Can you work these out from the drawing? Everything is in mm from the part's minimum corner. Give positions to 0.01 mm unless a question says otherwise; leave off trailing zeros. Order: outer loops, then holes, each group sorted by start corner. A loop starts at its lowest first (then second) coordinate and runs counter-clockwise, first axis right, second up. Notation, with made-up numbers: (-3, 83.5) - (43, 83.5) arc R21 ccw to (43, 103.5) - close; hole circle Ø5 at (36, 76.25). An arc over 180 degrees is marked (long way). One line per question, with ' | ' between items.
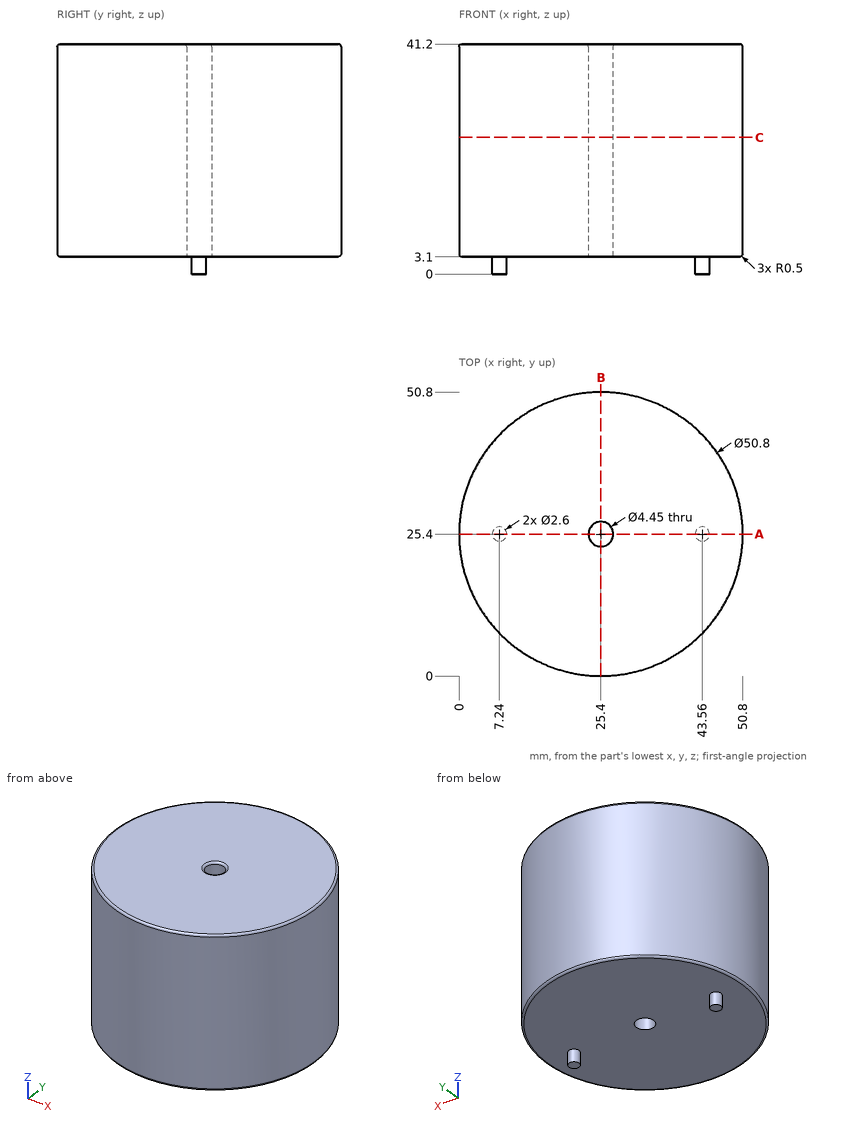
1) I'm going to push flat-ended pins straight in: P1, Ø10, axis at y = 14.5, z = 14.5, coming from the +X side; P2, Ø3, axis at x = 30, z = 9, coming from the +Y side; P3, Ø3, axis at x = 29.5, y = 34.5, coming from the -Z side. Where does each tip first touch, or does it pass through?
Model answer:
P1: stops at x = 50.11 | P2: stops at y = 50.61 | P3: stops at z = 3.1
2) Please list where these lines run through material, in increasing order: L1, parallel to Y at x = 25.4, z = 18.5 (3 decimals); L2, parallel to X at y = 25.5, z = 10; L3, parallel to Z at x = 4, y = 35.
Model answer:
L1: y = 0 to 23.175, 27.625 to 50.8 | L2: x = 0 to 23.18, 27.62 to 50.8 | L3: z = 3.1 to 41.2
3) I want a section at B-B (x = 25.4). List the corners of the cut face in (y, z) for me (3 decimals).
Model answer:
outline: (0, 3.6) arc R0.5 ccw to (0.5, 3.1) - (23.175, 3.1) - (23.175, 40.7) arc R0.5 ccw to (22.675, 41.2) - (0.5, 41.2) arc R0.5 ccw to (0, 40.7) - close; (27.625, 3.1) - (50.3, 3.1) arc R0.5 ccw to (50.8, 3.6) - (50.8, 40.7) arc R0.5 ccw to (50.3, 41.2) - (28.125, 41.2) arc R0.5 ccw to (27.625, 40.7) - close
4) I want a section at A-A (y = 25.4). List the corners of the cut face in (x, z) for me (3 decimals).
Model answer:
outline: (0, 3.6) arc R0.5 ccw to (0.5, 3.1) - (5.94, 3.1) - (5.94, 0) - (8.54, 0) - (8.54, 3.1) - (23.175, 3.1) - (23.175, 40.7) arc R0.5 ccw to (22.675, 41.2) - (0.5, 41.2) arc R0.5 ccw to (0, 40.7) - close; (27.625, 3.1) - (42.26, 3.1) - (42.26, 0) - (44.86, 0) - (44.86, 3.1) - (50.3, 3.1) arc R0.5 ccw to (50.8, 3.6) - (50.8, 40.7) arc R0.5 ccw to (50.3, 41.2) - (28.125, 41.2) arc R0.5 ccw to (27.625, 40.7) - close
5) I want a section at C-C (z = 24.5). List the corners of the cut face in (x, y) for me (3 decimals).
Model answer:
outline: circle Ø50.8 at (25.4, 25.4); hole circle Ø4.45 at (25.4, 25.4)
